from build123d import *

# Parameters (mm, degrees)
BASE_EXTRUSION_DEPTH    = 4
ESQUISSE2_R             = 3.3234375
ENL_V_MAT_EXTRU_1_DEPTH = 5


with BuildPart() as part:
    # Esquisse1 → Base-Extrusion (new body)
    with BuildSketch(Plane.XY):
        Polygon((-7.505553499, 0), (-3.75277675, 6.5), (3.75277675, 6.5), (7.505553499, 0), (3.75277675, -6.5), (-3.75277675, -6.5), align=None)
    extrude(amount=BASE_EXTRUSION_DEPTH)

    # Esquisse2 → Enlèv. mat.-Extru.1 (cut, through all)
    with BuildSketch(Plane.XY.offset(4)):
        Circle(ESQUISSE2_R)
    extrude(amount=-ENL_V_MAT_EXTRU_1_DEPTH, mode=Mode.SUBTRACT)

    # Esquisse3 → Enlever de la matière-Révolution1 (revolve, cut)
    with BuildSketch(Plane(origin=(0, 0, 0), x_dir=(1, 0, 0), z_dir=(0, 1, 0))):
        Polygon((-6.25, 0), (-7.505553499, 0), (-7.505553499, -0.724894151), align=None)
    enlever_de_la_mati_re_r_volution1 = revolve(axis=Axis((0, 0, 0), (0, 0, 1)), mode=Mode.SUBTRACT)

    # Symétrie1: Enlever de la matière-Révolution1 across Plan4
    add(enlever_de_la_mati_re_r_volution1.mirror(Plane(origin=(0, 0, 2), x_dir=(-1, 0, 0), z_dir=(0, 0, -1))), mode=Mode.SUBTRACT)


solid = part.part
For this review, take the finished solid that the model builds, in its own axes (mm). Give positions to 0.01 mm unless a question says otherwise; leave off trailing zeros. Loops run counter-clockwise (first coordinate to the right, second up) from the corner with the lowest first, then second, coordinate; pieces in that order, holes last. Notation, with made-up numbers: M 2.5,54.25 L 30.5,54.25 A27 cw 30.5,75.25 Z; hole C 71.5,-14.75 d10. An arc over 180 degrees is marked long. Answer as a JSON object with one key per item and string values. Group by question number.
Q1. Mouldability with a two-part tool opening along Y and no side actions: class faces 1 (the flat face through (5.66, -3.2, 1.97)), 2 (the cylindrical face through (-2.64, -2.02, 2.03)), 3 (the flat face through (-5.66, 3.2, 1.97)) as +Y half, -Y half, draft (parallel to the pull), parting line (faces both ways), or undercut.
Q2. Insertion check: P1, Ø1.5, axis at y = -2.5, z = 2.5, coming from the -X side; P2, Ø2, axis at x = -5, z = 1, coming from the +Y side; P3, Ø1, axis at x = 0, y = 3, coming from the -Z side. Each pin has a flat end and moves straight along its axis. Give the tip position at first contact, or say it passes through.
Q3. Add section A-A on z = 2.15. Give the boundary of the cut face in (x, y).
Q4. Add section B-B on x = 0. Give the boundary of the cut face in (y, z).
Q5. For probe 1 along Y at (x, z) = (0, 1.25); probe 2 along X at (y, z) = (-3, 3.15); probe 3 along Z at (x, y) = (-6, -2.5), list the stretches that pass through material, from the lowest coordinate up. Write a range as [from, to].
Checked values:
{
 "1": {"face 1": "-Y half", "face 2": "undercut", "face 3": "+Y half"},
 "2": {"P1": "x = -6.5", "P2": "y = 6.07", "P3": "z = 0"},
 "3": {"outline": "M -7.51,0 L -3.75,-6.5 L 3.75,-6.5 L 7.51,0 L 3.75,6.5 L -3.75,6.5 Z; hole C 0,0 d6.65"},
 "4": {"outline": "M -6.5,0.14 L -6.25,0 L -3.32,0 L -3.32,4 L -6.25,4 L -6.5,3.86 Z; M 3.32,0 L 6.25,0 L 6.5,0.14 L 6.5,3.86 L 6.25,4 L 3.32,4 Z"},
 "5": {"probe 1": "[-6.5, -3.32], [3.32, 6.5]", "probe 2": "[-5.77, -1.43], [1.43, 5.77]", "probe 3": "[0.14, 3.86]"}
}
